Input: part model. Units: mm. Frame: model coordinates. A direction names the side the tool comes from. Give positions to 0.01 mm unless a question says otherwise; leave off trailing zeros. Loops run counter-clockwise (first coordinate to the right, second up) from the corner with the lowest first, then second, coordinate; pieces in that order, holes last. Notation, with made-up numbers: (16.5, -16.5) - (67.5, -16.5) arc R31 cw to (67.5, 18.5) - close; hole circle Ø11 at (-28.5, 25). An arc over 180 degrees is marked (long way). Answer as a JSON object with one key per item and string values.
Autodesk Inventor part; units mm, degrees
ref_plane "YZ Plane" through (0, 0, 0) normal (1, 0, 0) x (0, 1, 0)
ref_plane "XZ Plane" through (0, 0, 0) normal (0, 1, 0) x (-1, 0, 0)
ref_plane "XY Plane" through (0, 0, 0) normal (0, 0, 1) x (1, 0, 0)
sketch "Sketch1" plane through (0, 0, 0) normal (1, 0, 0) x (0, 1, 0)
  circle A0 centre (0, 0) radius 2.54
  circle A1 centre (0, 0) radius 6.35
  line L0 (-6.35, 0) -> (-6.35, 12.7)
  line L1 (-6.35, 12.7) -> (21.7578, 32.3813)
  line L2 (21.7578, 32.3813) -> (25.4, 27.1797)
  line L3 (25.4, 27.1797) -> (25.4, 19.4278)
  line L4 (25.4, 19.4278) -> (6.35, 6.0888)
  line L5 (6.35, 0) -> (6.35, 6.0888)
  line L6 (23.2147, 30.3006) -> (-6.35, 9.5992)
  line L7 (6.35, 0) -> (6.35, 18.4919)
  line L8 (6.35, 18.4919) -> (4.8931, 20.5725)
  dimension "d0" = 5.08
  dimension "d1" = 12.7
  dimension "d2" = 12.7
  dimension "d3" = 145
  dimension "d5" = 125
  dimension "d6" = 31.75
  dimension "d7" = 12.7
  dimension "d8" = 6.35
  dimension "d15" = 2.54
extrude "Extrusion1" add sketch "Sketch1" along normal mid plane 25.4
extrude "Extrusion2" add sketch "Sketch1" along normal mid plane 30.48 contours A0
fillet "Fillet1" radius 4.7625 3 edges at (0, 25.4, 27.1797) (0, 21.7578, 32.3813) (0, 25.4, 19.4278)
fillet "Fillet2" radius 0.7937 4 edges at (15.24, -2.54, 0) (12.7, -2.54, 0) (-15.24, -2.54, 0) (-12.7, -2.54, 0)
extrude "Extrusion3" cut sketch "Sketch1" along normal mid plane 19.05 contours L7 L6 L2 L3 L4
extrude "Extrusion4" cut sketch "Sketch1" along normal mid plane 15.24 contours A0 | A1 | A1 L0 L6 L7 L5 | L0 L1 L8 L6
equation "\"d8\" = 0.5 * d7"
properties part number "LegV3"
Item 1: Cut plane C-C (y = 13). Return loops of the section in (x, z) (3 decimals), then the cut area to 3 significant figures.
Geometry check:
{"outline": "(-12.7, 10.745) - (-9.525, 10.745) - (-9.525, 23.148) - (9.525, 23.148) - (9.525, 10.745) - (12.7, 10.745) - (12.7, 26.249) - (-12.7, 26.249) - close", "area": "158 mm2"}
Item 2: Mould query, pull axis X, two halves, no side actions, for faces 4 (the face through (9, 6.35, 7)), 5 (the face through (12.7, 9, 12)), 6 (the face through (10, -6.35, 6)). Classes: released by +X, released by -X, zero draft, split by the parting line, or undercut.
Geometry check:
{"face 4": "undercut", "face 5": "released by +X", "face 6": "zero draft"}
Item 3: Cut plane A-A (z = 5). Return loops of the section in (x, y), then the cut area to 3 significant figures.
Geometry check:
{"outline": "(-12.7, -6.35) - (-7.62, -6.35) - (-7.62, 6.35) - (-12.7, 6.35) - close; (7.62, -6.35) - (12.7, -6.35) - (12.7, 6.35) - (7.62, 6.35) - close", "area": "129 mm2"}
Item 4: Access query for faces 1 (the face through (-0.11, 5.63, 19.52)), 2 (the face through (-0.133, 14.672, 24.319)), 3 (the face through (-13.96, -0.33, 2.52)). Directions: +Z, -Z, +X, -X, +Y, -Y. A direction counts if a zero-diameter tool reaches every point of the face in a straight line with its end or side. Return the directions, or none.
Geometry check:
{"face 1": "-Z, -Y", "face 2": "-Z, +Y", "face 3": "-X"}
Item 5: Cut plane B-B (y = 0). Return loops of the section in (x, z).
Geometry check:
{"outline": "(-15.24, -1.75) arc R0.79 ccw to (-14.45, -2.54) - (-13.49, -2.54) arc R0.79 cw to (-12.7, -3.33) - (-12.7, -6.35) - (-7.62, -6.35) - (-7.62, 17.15) - (-12.7, 17.15) - (-12.7, 3.33) arc R0.79 cw to (-13.49, 2.54) - (-14.45, 2.54) arc R0.79 ccw to (-15.24, 1.75) - close; (7.62, -6.35) - (12.7, -6.35) - (12.7, -3.33) arc R0.79 cw to (13.49, -2.54) - (14.45, -2.54) arc R0.79 ccw to (15.24, -1.75) - (15.24, 1.75) arc R0.79 ccw to (14.45, 2.54) - (13.49, 2.54) arc R0.79 cw to (12.7, 3.33) - (12.7, 17.15) - (7.62, 17.15) - close"}
Item 6: Contact query for flat-ended pins moving along their axis: P1, Ø1.5, axis at x = -10, z = 15, coming from the -Y side; P2, Ø4, axis at x = 10, z = 2, coming from the +Y side; P3, Ø9.5, axis at y = 14, z = 12, coming from the +X side. Output: stop coordinate, or through.
Geometry check:
{"P1": "stops at y = -4.14", "P2": "stops at y = 6.35", "P3": "stops at x = 12.7"}
Item 7: Material intervals for line 1 (X direction, y = 18, z = 20) (3 decimals); line 2 (X direction, y = 4, z = -3); line 3 (X direction, y = 12.5, z = 24), sorted ascending. Write a range as [from, to].
Geometry check:
{"line 1": "x = [-12.7, -9.525], [9.525, 12.7]", "line 2": "x = [-12.7, -7.62], [7.62, 12.7]", "line 3": "x = [-12.7, 12.7]"}
